from build123d import *

# Parameters (mm, degrees)
F3_D = 8
F5_D = 3.5


with BuildPart() as f1:
    # F0 (on Front) → F1 (revolve)
    with BuildSketch(Plane.XZ):
        Polygon((11.25, -0.01), (11.25, 3.49), (5.25, 3.49), (5.25, 13.49), (0, 13.49), (0, -1.51), (5.25, -1.51), (5.25, -0.01), align=None)
    revolve(axis=Axis((0, 0, 5.99), (0, 0, 1)))

    # F3 (through all)
    with Locations(Plane(origin=(0, 0, -1.51), x_dir=(1, 0, 0), z_dir=(0, 0, -1))):
        with Locations((0, 0)):
            Hole(F3_D / 2)

    # F5 (through all)
    with Locations(Plane(origin=(0, 0, -0.01), x_dir=(1, 0, 0), z_dir=(0, 0, -1))):
        with Locations((0, 8.5), (8.5, 0), (0, -8.5), (-8.5, 0)):
            Hole(F5_D / 2)


solid = f1.part
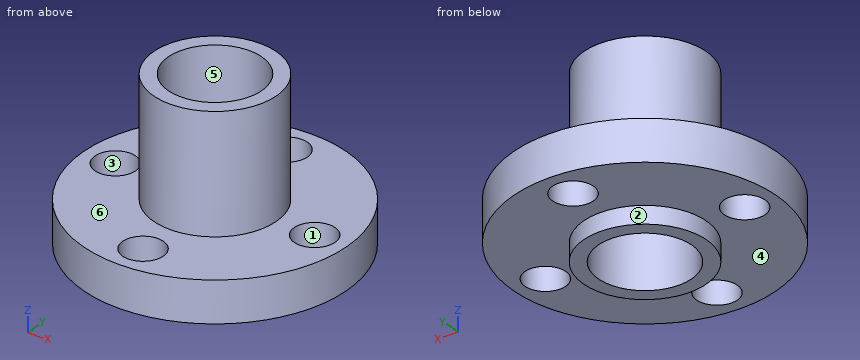
Verification items for the finished model (mm, model axes). Face numbers are marked on the shaded views. A direction names the side the tool comes from. Give positions to 0.01 mm unless a question says otherwise; leave off trailing zeros. Write each loop counter-clockwise with the first axis right and the second up, starting at its lowest first coordinate (ties: lowest second). Pieces come first, ordered by that corner, then holes.
(1) Cross-section at D-D (z = 12.25). Enter the section's corners in (x, y).
(2) Cross-section at C-C (z = 1.25). Enter the section's corners in (x, y), plus the area to 3 significant figures.
(3) Access from +Z, -Z, +X, -X, +Y, -Y to the whole of each face (thin tool, end or side, straight path). Record for the marked faces 5 and 6.
(4) Cross-section at B-B (x = -2.25). Enter the section's corners in (y, z), plus the area to 3 significant figures.
(5) Material ranges on line 1 (Y direction, x = 0, z = 2.35); line 2 (Y direction, x = -1.25, z = 2.75); line 3 (Y direction, x = 0, z = 10.25), recorded low to high.
(6) Mould release check, pull along X, two halves, no side actions. Record for the marked faces 1, 2, 3 and 4: +X half, -X half, draft (parallel to the pull), parting line (faces both ways), or undercut.
(7) Gauge pin test, flat ends, axial feed: pin 1 (3 mm diameter, centred on x = -7, z = 0.5, fed in from -Y); pin 2 (4 mm diameter, centred on x = -4.5, z = 2, fed in from -Y); pin 3 (4 mm diameter, centred on y = 6, z = 3, fed in from +X); pin 4 (12 mm diameter, centred on x = 8.5, y = 1.5, fed in from +Z). Record the tip position at first contact, or that the pin passes through.
(8) Cross-section at A-A (y = 0). Enter the section's corners in (x, z).
Worked out:
1. outline: circle Ø10.5 at (0, 0); hole circle Ø8 at (0, 0)
2. outline: circle Ø22.5 at (0, 0); hole circle Ø3.5 at (-8.5, 0); hole circle Ø8 at (0, 0); hole circle Ø3.5 at (0, -8.5); hole circle Ø3.5 at (0, 8.5); hole circle Ø3.5 at (8.5, 0)
2. area: 309 mm2
3. face 5: +Z, -Z
3. face 6: +Z
4. outline: (-11.02, -0.01) - (-4.74, -0.01) - (-4.74, -1.51) - (-3.31, -1.51) - (-3.31, 13.49) - (-4.74, 13.49) - (-4.74, 3.49) - (-11.02, 3.49) - close; (3.31, -1.51) - (4.74, -1.51) - (4.74, -0.01) - (11.02, -0.01) - (11.02, 3.49) - (4.74, 3.49) - (4.74, 13.49) - (3.31, 13.49) - close
4. area: 87.0 mm2
5. line 1: y = -11.25 to -10.25, -6.75 to -4, 4 to 6.75, 10.25 to 11.25
5. line 2: y = -11.18 to -9.72, -7.28 to -3.8, 3.8 to 7.28, 9.72 to 11.18
5. line 3: y = -5.25 to -4, 4 to 5.25
6. face 1: undercut
6. face 2: parting line
6. face 3: undercut
6. face 4: draft
7. pin 1: stops at y = -9.81
7. pin 2: stops at y = -10.97
7. pin 3: stops at x = 10.51
7. pin 4: stops at z = 13.49
8. outline: (-11.25, -0.01) - (-10.25, -0.01) - (-10.25, 3.49) - (-11.25, 3.49) - close; (-6.75, -0.01) - (-5.25, -0.01) - (-5.25, -1.51) - (-4, -1.51) - (-4, 13.49) - (-5.25, 13.49) - (-5.25, 3.49) - (-6.75, 3.49) - close; (4, -1.51) - (5.25, -1.51) - (5.25, -0.01) - (6.75, -0.01) - (6.75, 3.49) - (5.25, 3.49) - (5.25, 13.49) - (4, 13.49) - close; (10.25, -0.01) - (11.25, -0.01) - (11.25, 3.49) - (10.25, 3.49) - close
